Build history of the part. All positions in model axes, mm. Face numbers are marked on the shaded views. A direction names the side the tool comes from. Round coordinates to 2 decimals unless told otherwise and drop trailing zeros. Order: outer loops, then holes, each group sorted by start corner. A loop starts at its lowest first (then second) coordinate and runs counter-clockwise, first axis right, second up. Notation, with made-up numbers: (9.5, -26) -> (25.5, -26) arc R19 ccw to (25.5, 1) -> close; hole circle Ø5 at (-7, -35). An arc over 180 degrees is marked (long way). Answer as a JSON object with one key per item and string values.
from build123d import *

# Parameters (mm, degrees)
BOSS_EXTRUDE1_DEPTH = 1.5


with BuildPart() as part:
    # Sketch1 → Boss-Extrude1 (new body, symmetric)
    with BuildSketch(Plane.XY):
        with BuildLine():
            Line((1.5, -15), (6.25, -15))
            Line((6.25, -15), (6.25, 15))
            ThreePointArc((6.25, 15), (0, 21.25), (-6.25, 15))
            Line((-6.25, 15), (-6.25, -15))
            Line((-6.25, -15), (-1.5, -15))
            Line((-1.5, -15), (-1.5, 15))
            Line((-1.5, 15), (1.5, 15))
            Line((1.5, 15), (1.5, -15))
        make_face()
    extrude(amount=BOSS_EXTRUDE1_DEPTH, both=True)


solid = part.part
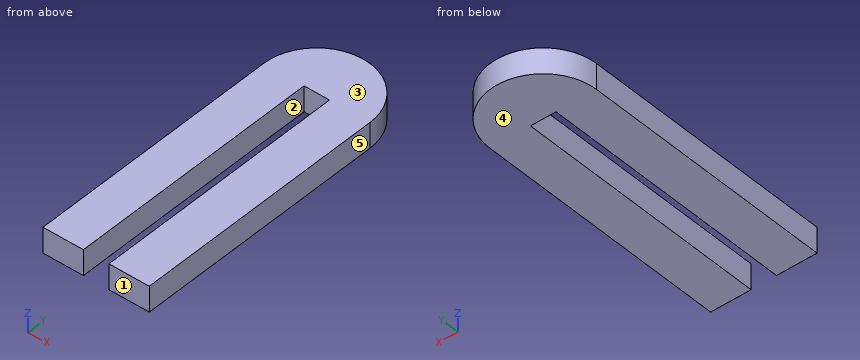
1) Cut at A-A, the plane z = -1. Give the cut face in (x, y), plus the area to 3 significant figures.
Checked values:
{"outline": "(-6.25, -15) -> (-1.5, -15) -> (-1.5, 15) -> (1.5, 15) -> (1.5, -15) -> (6.25, -15) -> (6.25, 15) arc R6.25 ccw to (-6.25, 15) -> close", "area": "346 mm²"}
2) Flat gauge pin, fed straight in: pin 1 Ø0.9 at (x, z) = (-0.5, 0.5) entering from -Y. Where does the tip first touch, or does it go through?
Checked values:
{"pin 1": "stops at y = 15"}
3) Pull direction Z, two halves, no side cores. Call the marked faces 3, 4 and 5: pulls with the +Z half, pulls with the -Z half, needs draft (parallel to the pull), parting line crosses it, or undercut.
Checked values:
{"face 3": "pulls with the +Z half", "face 4": "pulls with the -Z half", "face 5": "needs draft"}
4) Probe L1, parallel to X at y = -5, z = -0.2; L2, parallel to Y at x = 2.5, z = 1.15; L3, parallel to Y at x = 3, z = -0.3. List the from-to ranges inside material, lowest first. Write a range as from..to.
Checked values:
{"L1": "x = -6.25..-1.5, 1.5..6.25", "L2": "y = -15..20.73", "L3": "y = -15..20.48"}
5) Cut at C-C, the plane y = 17. Give the cut face in (x, z).
Checked values:
{"outline": "(-5.92, -1.5) -> (5.92, -1.5) -> (5.92, 1.5) -> (-5.92, 1.5) -> close"}
6) Cut at B-B, the plane x = 0. Give the cut face in (y, z).
Checked values:
{"outline": "(15, -1.5) -> (21.25, -1.5) -> (21.25, 1.5) -> (15, 1.5) -> close"}
7) Which spindle directions (+Z, -Z, +X, -X, +Y, -Y) get a long thin tool onto all of the face, cutting with end or side? Do the marked faces 1 and 2. Say none if no direction does.
Checked values:
{"face 1": "+Z, -Z, +X, -X, -Y", "face 2": "+Z, -Z, -Y"}
